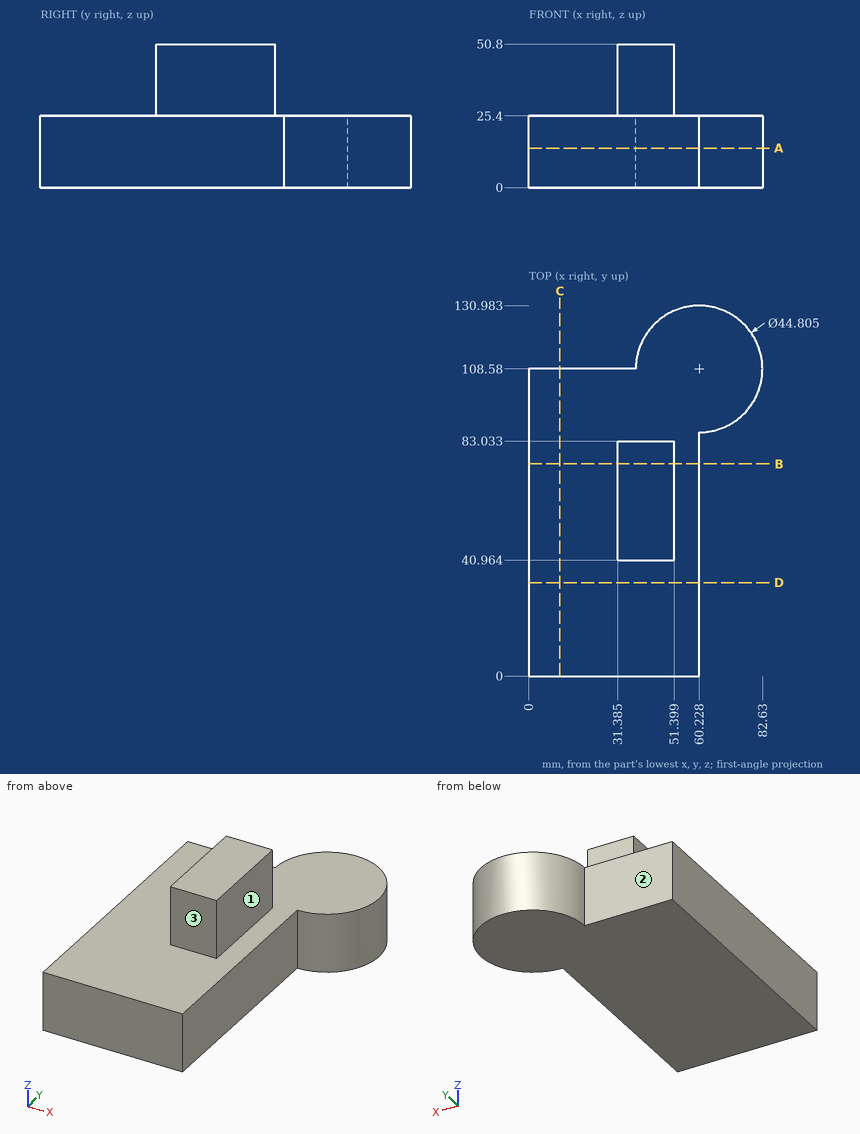
Part print with two shaded views. Sizes in mm from the minimum x, y, z corner. A direction names the side the tool comes from. Give positions to 0.01 mm unless a question says otherwise; leave off trailing zeros. Loops run counter-clockwise (first coordinate to the right, second up) from the corner with the lowest first, then second, coordinate; pieces in that order, holes last. Notation, with made-up numbers: (-4, 31.5) - (33, 31.5) arc R33 ccw to (33, 60.5) - close; hole circle Ø10 at (-37.75, 86.5). An arc over 180 degrees is marked (long way). Put each result on its own line as item: value.
Q1. Probe line 1 along X through (y, z) = (83.5, 23.5); line 2 along Z through (x, y) = (14, 42.5); line 3 along Y through (x, z) = (34, 32) (1 decimal). List the from-to ranges inside material, lowest first.
Filled in:
line 1: x = 0 to 60.23
line 2: z = 0 to 25.4
line 3: y = 41 to 83
Q2. Slice it at D-D (y = 33). Give the cut face in (x, z).
Filled in:
outline: (0, 0) - (60.23, 0) - (60.23, 25.4) - (0, 25.4) - close
Q3. Slice it at B-B (y = 75). Give the cut face in (x, z) (1 decimal).
Filled in:
outline: (0, 0) - (60.2, 0) - (60.2, 25.4) - (51.4, 25.4) - (51.4, 50.8) - (31.4, 50.8) - (31.4, 25.4) - (0, 25.4) - close
Q4. Slice it at C-C (x = 11). Give the cut face in (y, z).
Filled in:
outline: (0, 0) - (108.58, 0) - (108.58, 25.4) - (0, 25.4) - close
Q5. Flat gauge pins, fed straight in: pin 1 (12 mm diameter, centred on x = 30.5, z = 42.5, fed in from +Y); pin 2 (22 mm diameter, centred on x = 37.5, z = 32.5, fed in from -Y); pin 3 (2 mm diameter, centred on y = 89.5, z = 18, fed in from +X) (1 decimal); pin 4 (12 mm diameter, centred on y = 40, z = 21.5, fed in from +X). Where does each tip first touch, or does it go through?
Filled in:
pin 1: stops at y = 83.03
pin 2: stops at y = 0
pin 3: stops at x = 73.5
pin 4: stops at x = 60.23
Q6. Tool access for the marked faces 1, 2 and 3: list every direction of +Z, -Z, +X, -X, +Y, -Y with a clear straight run to the whole face (end or side of a thin tool).
Filled in:
face 1: +Z, +X, +Y, -Y
face 2: +Z, -Z, -X, +Y
face 3: +Z, +X, -X, -Y
Q7. Slice it at A-A (z = 14). Give the cut face in (x, y) (1 decimal), plus the area to 3 significant figures.
Filled in:
outline: (0, 0) - (60.2, 0) - (60.2, 86.2) arc R22.4 ccw (long way) to (37.8, 108.6) - (0, 108.6) - close
area: 7,720 mm²
